The model under review builds one solid part; all positions refer to its coordinate system, in mm. Give positions to 0.01 mm unless a question says otherwise; leave off trailing zeros. Write each loop counter-clockwise with the first axis right and the second up, starting at its lowest first coordinate (ties: lowest second). Pieces come first, ordered by that corner, then holes.
from build123d import *

# Parameters (mm, degrees)
SKETCH1_W           = 25.4
SKETCH1_H           = 12.7
SKETCH1_W_2         = 19.05
SKETCH1_H_2         = 6.35
BOSS_EXTRUDE1_DEPTH = 520.7
SKETCH2_R           = 3.3528
CUT_EXTRUDE1_DEPTH  = 13.7


with BuildPart() as part:
    # Sketch1 → Boss-Extrude1 (new body)
    with BuildSketch(Plane(origin=(0, 0, 0), x_dir=(0, 0, -1), z_dir=(1, 0, 0))):
        with Locations((12.7, 6.35)):
            Rectangle(SKETCH1_W, SKETCH1_H)
        with Locations((12.7, 6.35)):
            Rectangle(SKETCH1_W_2, SKETCH1_H_2, mode=Mode.SUBTRACT)
    extrude(amount=BOSS_EXTRUDE1_DEPTH)

    # Sketch2 → Cut-Extrude1 (cut, through all)
    with BuildSketch(Plane(origin=(0, 12.7, 0), x_dir=(1, 0, 0), z_dir=(0, 1, 0))):
        with Locations((6.35, 12.7)):
            Circle(SKETCH2_R)
        with Locations((514.35, 12.7)):
            Circle(SKETCH2_R)
    extrude(amount=-CUT_EXTRUDE1_DEPTH, mode=Mode.SUBTRACT)


solid = part.part
1) To check wall thickness, follow probe 1 along X at (y, z) = (1.05, -12.7); probe 2 along Y at (x, z) = (470, -14.75) (3 decimals); probe 3 along Z at (x, y) = (483, 6) (3 decimals). State the ranges of each line that lie inside material, in increasing order.
2) Consider section A-A, the plane x = 408. Give the boundary of the cut face in (y, z) (3 decimals).
3) Consider section B-B, the plane y = 7.25. Give the boundary of the cut face in (x, z) (3 decimals).
4) The part is to be moulded in two halves that separate along Y. For faces 1 (the flat face through (257, 12.7, -13)), 2 (the flat face through (257, 9.525, -13)), 3 (the flat face through (257, 3.175, -13)), 4 (the flat face through (257, 6, 0)), say which applies: +Y half, -Y half, draft (parallel to the pull), parting line (faces both ways), or undercut.
5) Insertion check: pin 1 (2 mm diameter, centred on y = 8, z = -13.5, fed in from +X). The pin has a flat end and moves straight along its axis. Give the tip position at first contact, or say it passes through.
Answer block:
1. probe 1: x = 0 to 3, 9.7 to 511, 517.7 to 520.7
1. probe 2: y = 0 to 3.175, 9.525 to 12.7
1. probe 3: z = -25.4 to -22.225, -3.175 to 0
2. outline: (0, -25.4) - (12.7, -25.4) - (12.7, 0) - (0, 0) - close; hole (3.175, -22.225) - (9.525, -22.225) - (9.525, -3.175) - (3.175, -3.175) - close
3. outline: (0, -25.4) - (520.7, -25.4) - (520.7, -22.225) - (0, -22.225) - close; (0, -3.175) - (520.7, -3.175) - (520.7, 0) - (0, 0) - close
4. face 1: +Y half
4. face 2: undercut
4. face 3: undercut
4. face 4: draft
5. pin 1: passes through
